from build123d import *

# Parameters (mm, degrees)
F0_W     = 57.15
F0_H     = 85.09
F1_DEPTH = 63.5
F2_R     = 12.7
F3_DEPTH = 44.45
F4_R     = 7.62
F5_DEPTH = 25.4
F6_DEPTH = 57.151


with BuildPart() as f1:
    # F0 (on Right) → F1 (new body, symmetric)
    with BuildSketch(Plane.YZ):
        with Locations((28.575, 42.545)):
            Rectangle(F0_W, F0_H)
    extrude(amount=F1_DEPTH, both=True)

    # F2 (on Front) → F3 (cut)
    with BuildSketch(Plane.XZ):
        with BuildLine():
            Line((-63.5, 85.09), (-63.5, 34.29))
            Line((-63.5, 34.29), (-47.625, 34.29))
            Line((-47.625, 34.29), (-21.093426, 73.840173))
            ThreePointArc((-21.093426, 73.840173), (-11.952941, 82.101765), (0, 85.09))
            Line((0, 85.09), (-63.5, 85.09))
        make_face()
        with BuildLine():
            Line((47.625, 34.29), (63.5, 34.29))
            Line((63.5, 34.29), (63.5, 85.09))
            Line((63.5, 85.09), (0, 85.09))
            ThreePointArc((0, 85.09), (11.952941, 82.101765), (21.093426, 73.840173))
            Line((21.093426, 73.840173), (47.625, 34.29))
        make_face()
        with Locations((0, 59.69)):
            Circle(F2_R)
    extrude(amount=-F3_DEPTH, mode=Mode.SUBTRACT)

    # F4 (on face) → F5 (cut)
    with BuildSketch(Plane.XY.offset(85.09)):
        with Locations((0, 22.225)):
            Circle(F4_R)
    extrude(amount=-F5_DEPTH, mode=Mode.SUBTRACT)

    # F2 (on Front) → F6 (cut, through all)
    with BuildSketch(Plane.XZ):
        Polygon((-63.5, 0), (-31.75, 0), (-31.75, 12.7), (-12.7, 12.7), (-12.7, 21.59), (-63.5, 21.59), align=None)
        Polygon((44.45, 12.7), (44.45, 0), (63.5, 0), (63.5, 21.59), (12.7, 21.59), (12.7, 12.7), align=None)
    extrude(amount=-F6_DEPTH, mode=Mode.SUBTRACT)


solid = f1.part
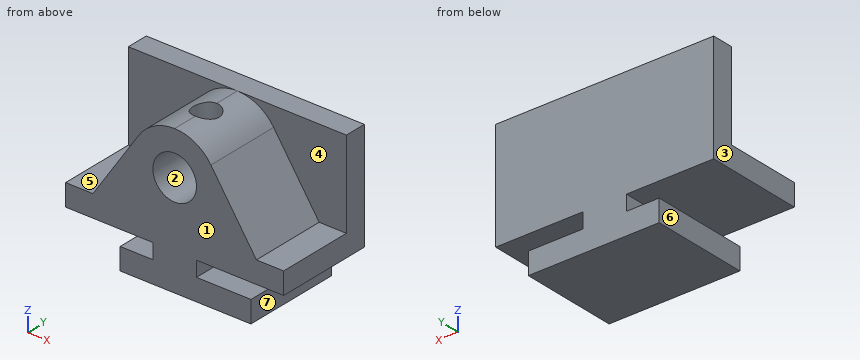
Here's how the part is built. I have some questions about the finished solid (model axes, mm). Face numbers are marked on the shaded views. A direction names the side the tool comes from. Round coordinates to 2 decimals unless told otherwise and drop trailing zeros. Order: outer loops, then holes, each group sorted by start corner. A loop starts at its lowest first (then second) coordinate and runs counter-clockwise, first axis right, second up. Notation, with made-up numbers: M 50,46.25 L 95,46.25 A22 ccw 95,52.25 Z; hole C 46.25,-21 d8. An arc over 180 degrees is marked long. Return JSON: item names as keys, results as strings. Group by question number.
1. On a 3-axis mill with a long thin cutter (end or side, diameter ignored), from which of +Z, -Z, +X, -X, +Y, -Y can I reach the whole of each face in a straight line? I mean the marked faces 4, 5, 6 and 7. Say none if no direction works.
2. If we section it at A-A on y = 39.5: List the corners of the cut face in (x, z) for me (3 decimals).
3. I'm going to push flat-ended pins straight in: pin 1 Ø5 at (x, y) = (54.5, 16.5) entering from +Z; pin 2 Ø2 at (x, y) = (32.5, 40) entering from +Z; pin 3 Ø7 at (y, z) = (28, 16) entering from -X. Where does each tip first touch, or does it pass through?
4. If we section it at D-D on y = 46.5: List the corners of the cut face in (x, z) for me.
5. If we mould it in two halves opening along X, with no side actions, what happens to the marked faces 1, 2 and 3? For each: pulls with the +X half, pulls with the -X half, needs draft (parallel to the pull), parting line crosses it, or undercut.
6. Please list where these lines run through material, in increasing order: probe 1 along Z at (x, y) = (0, 11.5); probe 2 along Y at (x, z) = (0, 74.75) (3 decimals); probe 3 along Z at (x, y) = (42, 54).
7. If we section it at B-B on x = -16: List the corners of the cut face in (y, z) for me, then the cut area to 3 significant figures.
8. If we section it at C-C on x = -54.5: List the corners of the cut face in (y, z) for me.
Reply:
{
 "1": {"face 4": "+Z, +X, -Y", "face 5": "+Z, -X, -Y", "face 6": "-Z, -X, +Y, -Y", "face 7": "-Z, +X, +Y, -Y"},
 "2": {"outline": "M -63.5,21.59 L -12.7,21.59 L -12.7,12.7 L -31.75,12.7 L -31.75,0 L 44.45,0 L 44.45,12.7 L 12.7,12.7 L 12.7,21.59 L 63.5,21.59 L 63.5,34.29 L 47.625,34.29 L 21.093,73.84 A25.4 ccw -21.093,73.84 L -47.625,34.29 L -63.5,34.29 Z; hole C 0,59.69 d25.4"},
 "3": {"pin 1": "z = 34.29", "pin 2": "z = 58.33", "pin 3": "x = -31.75"},
 "4": {"outline": "M -63.5,21.59 L -12.7,21.59 L -12.7,12.7 L -31.75,12.7 L -31.75,0 L 44.45,0 L 44.45,12.7 L 12.7,12.7 L 12.7,21.59 L 63.5,21.59 L 63.5,85.09 L -63.5,85.09 Z"},
 "5": {"face 1": "needs draft", "face 2": "undercut", "face 3": "pulls with the -X half"},
 "6": {"probe 1": "0 to 46.99, 72.39 to 85.09", "probe 2": "0 to 14.605, 29.845 to 57.15", "probe 3": "0 to 12.7, 21.59 to 85.09"},
 "7": {"outline": "M 0,0 L 57.15,0 L 57.15,12.7 L 0,12.7 Z; M 0,21.59 L 57.15,21.59 L 57.15,85.09 L 44.45,85.09 L 44.45,79.42 L 0,79.42 Z", "area": "4,100 mm^2"},
 "8": {"outline": "M 0,21.59 L 57.15,21.59 L 57.15,85.09 L 44.45,85.09 L 44.45,34.29 L 0,34.29 Z"}
}
